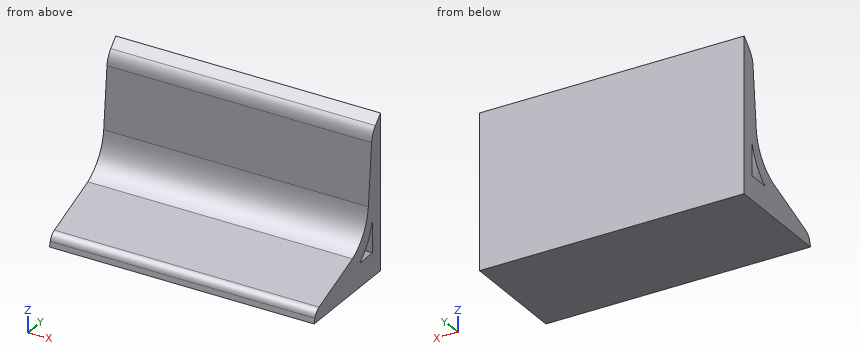
from build123d import *

# Parameters (mm, degrees)
CROQUIS1_W              = 120
CROQUIS1_H              = 50
SALIENTE_EXTRUIR1_DEPTH = 70
CORTAR_EXTRUIR1_DEPTH   = 121


with BuildPart() as part:
    # Croquis1 → Saliente-Extruir1 (new body)
    with BuildSketch(Plane.XY):
        with Locations((200.700947131, 43.628006873)):
            Rectangle(CROQUIS1_W, CROQUIS1_H)
    extrude(amount=SALIENTE_EXTRUIR1_DEPTH)

    # Croquis2 → Cortar-Extruir1 (cut)
    with BuildSketch(Plane(origin=(260.700947131, 0, 0), x_dir=(0, 0, -1), z_dir=(1, 0, 0))):
        with BuildLine():
            Line((-70, 68.628006873), (-66.203930164, 64.831937037))
            ThreePointArc((-66.203930164, 64.831937037), (-63.370887429, 62.845458633), (-60.030458687, 61.943370276))
            Line((-60.030458687, 61.943370276), (-32.714126266, 59.481528961))
            ThreePointArc((-32.714126266, 59.481528961), (-22.428502516, 55.786756469), (-15.255184219, 47.541218021))
            Line((-15.255184219, 47.541218021), (-5.740714687, 22.291279647))
            ThreePointArc((-5.740714687, 22.291279647), (-4.393024365, 20.325605767), (-2.288474759, 19.207118412))
            Line((-2.288474759, 19.207118412), (0, 18.628006873))
            Line((0, 18.628006873), (-70, 18.628006873))
            Line((-70, 18.628006873), (-70, 68.628006873))
        make_face()
        with BuildLine():
            Line((-10.777042467, 52.920195468), (-10.777042467, 62.571113796))
            Line((-10.777042467, 62.571113796), (-24.848704029, 62.571113796))
            ThreePointArc((-24.848704029, 62.571113796), (-16.959352467, 58.990142997), (-10.777042467, 52.920195468))
        make_face()
    extrude(amount=-CORTAR_EXTRUIR1_DEPTH, mode=Mode.SUBTRACT)


solid = part.part
The model under review builds one solid part; all positions refer to its coordinate system, in mm. Round coordinates to 2 decimals unless told otherwise and drop trailing zeros. Write each loop counter-clockwise with the first axis right and the second up, starting at its lowest first coordinate (ties: lowest second). Pieces come first, ordered by that corner, then holes. Notation, with made-up numbers: (4.25, 25) - (14.25, 25) arc R11 ccw to (14.25, 38) - close; hole circle Ø9 at (-25, 35.5). An arc over 180 degrees is marked (long way). One line per item, written item: value. Start each with the question number.
1. To check wall thickness, follow L1, parallel to Z at x = 212.5, y = 55; L2, parallel to Y at x = 149, z = 48.5; L3, parallel to Y at x = 148.5, z = 39. State the ranges of each line that lie inside material, in increasing order. Write a range as from..to.
2. Consider section C-C on y = 33. Write out the cut boundary in (x, z), and give its area (3 significant figures).
3. Clearance check with flat-ended pins moving along their axes: P1, Ø8, axis at x = 157, y = 44, coming from the +Z side; P2, Ø1.5, axis at x = 171, y = 56, coming from the -Z side; P3, Ø7.5, axis at x = 192, y = 59.5, coming from the +Z side; P4, Ø6, axis at x = 225.5, z = 21, coming from the -Y side. State where each tip first meets the part, or that it passes through.
4. Consider section B-B on z = 42.5. Write out the cut boundary in (x, y), and give its area (3 significant figures).
5. Consider section A-A on x = 218.5. Write out the cut boundary in (y, z).
Checks:
1. L1: z = 0..10.78, 12.43..21.35
1. L2: y = 60.9..68.63
1. L3: y = 60.05..68.63
2. outline: (140.7, 0) - (260.7, 0) - (260.7, 9.78) - (140.7, 9.78) - close
2. area: 1,170 mm^2
3. P1: stops at z = 15.49
3. P2: stops at z = 0
3. P3: stops at z = 64.15
3. P4: stops at y = 51.76
4. outline: (140.7, 60.36) - (260.7, 60.36) - (260.7, 68.63) - (140.7, 68.63) - close
4. area: 992 mm^2
5. outline: (18.63, 0) - (68.63, 0) - (68.63, 70) - (64.83, 66.2) arc R10 ccw to (61.94, 60.03) - (59.48, 32.71) arc R21.67 cw to (47.54, 15.26) - (22.29, 5.74) arc R5 ccw to (19.21, 2.29) - close; hole (52.92, 10.78) - (62.57, 10.78) - (62.57, 24.85) arc R24.87 cw to start
